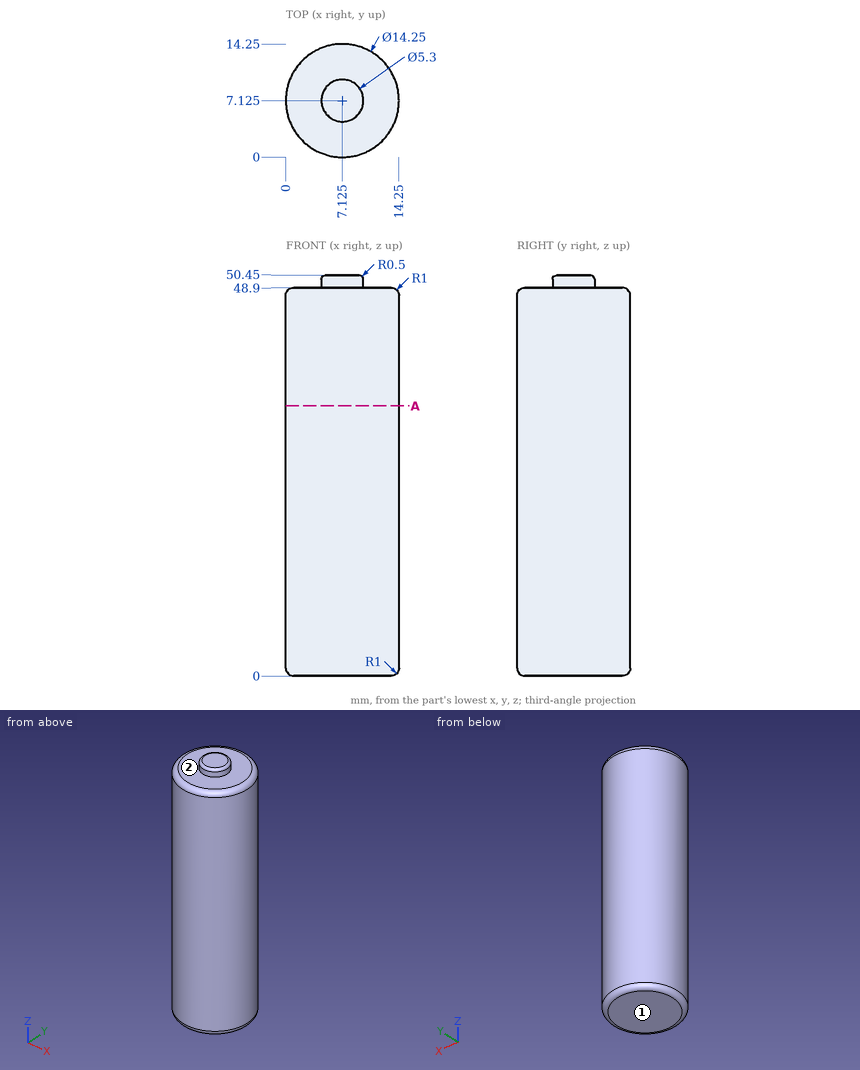
Could you check a few things on this drawing? It's one solid part, dimensions in mm from its lowest x, y, z. A direction names the side the tool comes from. Coordinates: 2 decimals unless noted, no trailing zeros. Loops run counter-clockwise (first coordinate to the right, second up) from the corner with the lowest first, then second, coordinate; pieces in that order, holes last. Notation, with made-up numbers: (65, -27) - (114, -27) arc R21 ccw to (114, -8) - close; hole circle Ø1 at (3, -38.5). An arc over 180 degrees is marked (long way). Answer as a JSON object with one key per item and string values. Group by question number.
Item 1: For pin 1 (4 mm diameter, centred on y = 1.5, z = 21, fed in from +X); pin 2 (2 mm diameter, centred on y = 11, z = 24, fed in from +X), each with a flat end and sliding along its axis, tell me the tip position at first contact or that it passes through.
Item 2: If we section it at A-A (z = 34): List the corners of the cut face in (x, y) for me (3 decimals), plus the area to 3 significant figures.
Item 3: On a 3-axis mill with a long thin cutter (end or side, diameter ignored), from which of +Z, -Z, +X, -X, +Y, -Y can I reach the whole of each face in a straight line? I mean the marked faces 1 and 2. Say none if no direction works.
Item 4: If I drill on L1, parallel to Z at x = 8, y = 9.75; L2, parallel to Y at x = 7, z = 35; L3, parallel to X at y = 6.75, z = 7, over which ranges is the centre line in solid material (lowest first)? Write a range as from..to.
Returned:
{
 "1": {"pin 1": "stops at x = 13.26", "pin 2": "stops at x = 13.64"},
 "2": {"outline": "circle Ø14.25 at (7.125, 7.125)", "area": "159 mm²"},
 "3": {"face 1": "-Z, +X, -X, +Y, -Y", "face 2": "+Z"},
 "4": {"L1": "z = 0..48.9", "L2": "y = 0..14.25", "L3": "x = 0.01..14.24"}
}
